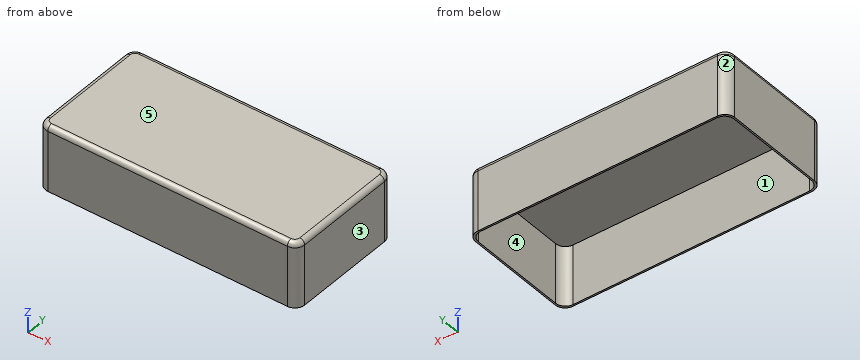
from build123d import *

# Parameters (mm, degrees)
PAD_DEPTH    = 20.07
POCKET_DEPTH = 18.42
FILLET_R     = 1.5


with BuildPart() as part:
    # Sketch → Pad (new body)
    with BuildSketch(Plane.XY):
        with BuildLine():
            Line((18.834122, 40.018788), (92.644122, 40.018788))
            ThreePointArc((95.644122, 37.018788), (94.765442, 39.140108), (92.644122, 40.018788))
            Line((95.644122, 37.018788), (95.644122, 5.428788))
            ThreePointArc((92.644122, 2.428788), (94.765442, 3.307467), (95.644122, 5.428788))
            Line((92.644122, 2.428788), (18.834122, 2.428788))
            ThreePointArc((15.834122, 5.428788), (16.712801, 3.307467), (18.834122, 2.428788))
            Line((15.834122, 5.428788), (15.834122, 37.018788))
            ThreePointArc((18.834122, 40.018788), (16.712801, 39.140108), (15.834122, 37.018788))
        make_face()
    extrude(amount=PAD_DEPTH)

    # Sketch001 (on Face9 of Pad) → Pocket (cut)
    with BuildSketch(Plane(origin=(0, 0, 0), x_dir=(1, 0, 0), z_dir=(0, 0, -1))):
        with BuildLine():
            Line((19.344122, -2.933788), (92.134122, -2.933788))
            ThreePointArc((95.134122, -5.933788), (94.255442, -3.812467), (92.134122, -2.933788))
            Line((95.134122, -5.933788), (95.134122, -36.513788))
            ThreePointArc((92.134122, -39.513788), (94.255442, -38.635108), (95.134122, -36.513788))
            Line((92.134122, -39.513788), (19.344122, -39.513788))
            ThreePointArc((16.344122, -36.513788), (17.222801, -38.635108), (19.344122, -39.513788))
            Line((16.344122, -36.513788), (16.344122, -5.933788))
            ThreePointArc((19.344122, -2.933788), (17.222801, -3.812467), (16.344122, -5.933788))
        make_face()
    extrude(amount=-POCKET_DEPTH, mode=Mode.SUBTRACT)

    # Fillet
    fillet_edges = [part.edges().sort_by_distance(p)[0] for p in [
        (15.834122, 21.223788, 20.07),
        (16.712801, 39.140108, 20.07),
        (55.739122, 40.018788, 20.07),
        (94.765442, 39.140108, 20.07),
        (95.644122, 21.223788, 20.07),
        (94.765442, 3.307467, 20.07),
        (55.739122, 2.428788, 20.07),
        (16.712801, 3.307467, 20.07),
    ]]
    fillet(fillet_edges, radius=FILLET_R)


solid = part.part
Check sheet for the modelled part. Datum: model origin and axes. Units: mm. Face numbers are marked on the shaded views. A direction names the side the tool comes from. Give positions to 0.01 mm unless a question says otherwise; leave off trailing zeros. Loops run counter-clockwise (first coordinate to the right, second up) from the corner with the lowest first, then second, coordinate; pieces in that order, holes last. Notation, with made-up numbers: M 49.5,-38.75 L 66.5,-38.75 A20 cw 66.5,-26.75 Z; hole C 42.25,81.5 d11. An arc over 180 degrees is marked long. Answer as a JSON object with one key per item and string values. Group by question number.
Q1. Go/stop test with a flat-tipped pin: P1, Ø6, axis at x = 56.5, y = 12, coming from the -Z side. Record where the tip stops, or that it passes through.
Q2. Release check for a two-part mould opening along Y. For the marked faces 1, 2 and 3 record: released by +Y, released by -Y, zero draft, split by the parting line, or undercut.
Q3. Cross-section at B-B on y = 15.5. Record the cut outline in (x, z).
Q4. Material ranges on line 1 along Y through (x, z) = (28, 10); line 2 along X through (y, z) = (23, 3); line 3 along Z through (x, y) = (76, 17), recorded low to high. Write a range as [from, to].
Q5. Access from +Z, -Z, +X, -X, +Y, -Y to the whole of each face (thin tool, end or side, straight path). Record for the marked faces 4 and 5.
Q6. Cross-section at A-A on z = 12.25. Record the cut outline in (x, y).
Q7. Cross-section at C-C on x = 50. Record the cut outline in (y, z), then the cut area to 3 significant figures.
Evaluation:
{
 "1": {"P1": "stops at z = 18.42"},
 "2": {"face 1": "undercut", "face 2": "released by +Y", "face 3": "zero draft"},
 "3": {"outline": "M 15.83,0 L 16.34,0 L 16.34,18.42 L 95.13,18.42 L 95.13,0 L 95.64,0 L 95.64,18.57 A1.5 ccw 94.14,20.07 L 17.33,20.07 A1.5 ccw 15.83,18.57 Z"},
 "4": {"line 1": "y = [2.43, 2.93], [39.51, 40.02]", "line 2": "x = [15.83, 16.34], [95.13, 95.64]", "line 3": "z = [18.42, 20.07]"},
 "5": {"face 4": "-Z", "face 5": "+Z, +X, -X, +Y, -Y"},
 "6": {"outline": "M 15.83,5.43 A3 ccw 18.83,2.43 L 92.64,2.43 A3 ccw 95.64,5.43 L 95.64,37.02 A3 ccw 92.64,40.02 L 18.83,40.02 A3 ccw 15.83,37.02 Z; hole M 16.34,5.93 A3 ccw 19.34,2.93 L 92.13,2.93 A3 ccw 95.13,5.93 L 95.13,36.51 A3 ccw 92.13,39.51 L 19.34,39.51 A3 ccw 16.34,36.51 Z"},
 "7": {"outline": "M 2.43,0 L 2.93,0 L 2.93,18.42 L 39.51,18.42 L 39.51,0 L 40.02,0 L 40.02,18.57 A1.5 ccw 38.52,20.07 L 3.93,20.07 A1.5 ccw 2.43,18.57 Z", "area": "79.7 mm2"}
}
